```python
from build123d import *

# Parameters (mm, degrees)
SKETCH1_W                    = 42.3
SKETCH1_H                    = 42.3
BOSS_EXTRUDE1_DEPTH          = 23.5
FILLET1_R                    = 4
SKETCH2_R                    = 1.5
CUT_EXTRUDE1_DEPTH           = 5
CHAMFER1_SIZE                = 1
CIRPATTERN1_COUNT            = 4
CHAMFER1_OF_CIRPATTERN1_SIZE = 1
SKETCH3_R                    = 11
BOSS_EXTRUDE2_DEPTH          = 2
SKETCH4_R                    = 2.5
BOSS_EXTRUDE3_DEPTH          = 20
FILLET2_R                    = 1
SKETCH5_W                    = 6
SKETCH5_H                    = 16.2
BOSS_EXTRUDE4_DEPTH          = 1
SKETCH6_W                    = 1
SKETCH6_H                    = 1
BOSS_EXTRUDE5_DEPTH          = 4.5
SKETCH7_W                    = 4
SKETCH7_H                    = 4
CUT_EXTRUDE2_DEPTH           = 18


with BuildPart() as part:
    # Sketch1 → Boss-Extrude1 (new body)
    with BuildSketch(Plane.XY):
        Rectangle(SKETCH1_W, SKETCH1_H)
    extrude(amount=BOSS_EXTRUDE1_DEPTH)

    # Fillet1
    fillet1_edges = [part.edges().sort_by_distance(p)[0] for p in [
        (-21.15, 21.15, 11.75),
        (21.15, 21.15, 11.75),
        (21.15, -21.15, 11.75),
        (-21.15, -21.15, 11.75),
    ]]
    fillet(fillet1_edges, radius=FILLET1_R)

    # Sketch2 → Cut-Extrude1 (cut)
    with BuildSketch(Plane.XY.offset(23.5)):
        with Locations((-15.5, -15.5)):
            Circle(SKETCH2_R)
    cut_extrude1 = extrude(amount=-CUT_EXTRUDE1_DEPTH, mode=Mode.SUBTRACT)

    # Chamfer1
    chamfer1_edges = [part.edges().sort_by_distance(p)[0] for p in [
        (-17, -15.5, 23.5),
    ]]
    chamfer(chamfer1_edges, length=CHAMFER1_SIZE)

    # CirPattern1: Cut-Extrude1 ×4 about axis
    cirpattern1_axis = Axis((0, 0, 0), (0, 0, 1))
    for i in range(1, CIRPATTERN1_COUNT):
        add(cut_extrude1.rotate(cirpattern1_axis, i * 360 / CIRPATTERN1_COUNT), mode=Mode.SUBTRACT)

    # Chamfer1 of CirPattern1
    chamfer1_of_cirpattern1_edges = [part.edges().sort_by_distance(p)[0] for p in [
        (15.5, -17, 23.5),
        (17, 15.5, 23.5),
        (-15.5, 17, 23.5),
    ]]
    chamfer(chamfer1_of_cirpattern1_edges, length=CHAMFER1_OF_CIRPATTERN1_SIZE)

    # Sketch3 → Boss-Extrude2 (add)
    with BuildSketch(Plane.XY.offset(23.5)):
        Circle(SKETCH3_R)
    extrude(amount=BOSS_EXTRUDE2_DEPTH)

    # Sketch4 → Boss-Extrude3 (add)
    with BuildSketch(Plane.XY.offset(25.5)):
        Circle(SKETCH4_R)
    extrude(amount=BOSS_EXTRUDE3_DEPTH)

    # Fillet2
    fillet2_edges = [part.edges().sort_by_distance(p)[0] for p in [
        (-21.15, 0, 0),
        (-21.15, 0, 23.5),
        (0, 21.15, 0),
        (21.15, 0, 0),
        (0, -21.15, 0),
        (-19.978427125, -19.978427125, 0),
        (19.978427125, -19.978427125, 0),
        (19.978427125, 19.978427125, 0),
        (-19.978427125, 19.978427125, 0),
        (0, 21.15, 23.5),
        (0, -21.15, 23.5),
        (21.15, 0, 23.5),
        (-19.978427125, -19.978427125, 23.5),
        (19.978427125, -19.978427125, 23.5),
        (19.978427125, 19.978427125, 23.5),
        (-19.978427125, 19.978427125, 23.5),
        (-11, 0, 25.5),
        (-2.5, 0, 45.5),
    ]]
    fillet(fillet2_edges, radius=FILLET2_R)

    # Sketch5 → Boss-Extrude4 (add)
    with BuildSketch(Plane(origin=(21.15, 0, 0), x_dir=(0, 0, -1), z_dir=(1, 0, 0))):
        with Locations((-6.2, 0)):
            Rectangle(SKETCH5_W, SKETCH5_H)
    extrude(amount=BOSS_EXTRUDE4_DEPTH)

    # Sketch6 → Boss-Extrude5 (add)
    with BuildSketch(Plane(origin=(22.15, 0, 0), x_dir=(0, 0, -1), z_dir=(1, 0, 0))):
        Polygon((-9.2, -7.1), (-4.2, -7.1), (-4.2, 7.1), (-9.2, 7.1), (-9.2, 8.1), (-3.2, 8.1), (-3.2, -8.1), (-9.2, -8.1), align=None)
        with Locations((-6.7, -4.26)):
            Rectangle(SKETCH6_W, SKETCH6_H)
        with Locations((-6.7, 1.42)):
            Rectangle(SKETCH6_W, SKETCH6_H)
        with Locations((-6.7, 4.26)):
            Rectangle(SKETCH6_W, SKETCH6_H)
        with Locations((-6.7, -1.42)):
            Rectangle(SKETCH6_W, SKETCH6_H)
    extrude(amount=BOSS_EXTRUDE5_DEPTH)

    # Sketch7 → Cut-Extrude2 (cut)
    with BuildSketch(Plane.XY.offset(45.5)):
        with Locations((-3.5, 0)):
            Rectangle(SKETCH7_W, SKETCH7_H)
    extrude(amount=-CUT_EXTRUDE2_DEPTH, mode=Mode.SUBTRACT)


solid = part.part
```
Read the model definition and answer for the solid it produces. Units are mm, in the model's axes. A direction names the side the tool comes from. Coordinates: 2 decimals unless noted, no trailing zeros. Write each loop counter-clockwise with the first axis right and the second up, starting at its lowest first coordinate (ties: lowest second). Pieces come first, ordered by that corner, then holes. Notation, with made-up numbers: (5.5, 44) -> (23.5, 44) arc R20 ccw to (23.5, 58) -> close; hole circle Ø8 at (15.25, 44). An arc over 180 degrees is marked (long way). Answer as a JSON object with one key per item and string values.
Q1. The part is cut by section A-A on z = 21. Give the vertices of the cut face in (x, y), then the cut area to 3 significant figures.
The answers:
{"outline": "(-21.15, -17.15) arc R4 ccw to (-17.15, -21.15) -> (17.15, -21.15) arc R4 ccw to (21.15, -17.15) -> (21.15, 17.15) arc R4 ccw to (17.15, 21.15) -> (-17.15, 21.15) arc R4 ccw to (-21.15, 17.15) -> close; hole circle Ø3 at (-15.5, -15.5); hole circle Ø3 at (-15.5, 15.5); hole circle Ø3 at (15.5, -15.5); hole circle Ø3 at (15.5, 15.5)", "area": "1,750 mm2"}
Q2. The part is cut by section B-B on x = -15.5. Give the vertices of the cut face in (y, z).
The answers:
{"outline": "(-21.15, 1) arc R1 ccw to (-20.15, 0) -> (20.15, 0) arc R1 ccw to (21.15, 1) -> (21.15, 22.5) arc R1 ccw to (20.15, 23.5) -> (18, 23.5) -> (17, 22.5) -> (17, 18.5) -> (14, 18.5) -> (14, 22.5) -> (13, 23.5) -> (-13, 23.5) -> (-14, 22.5) -> (-14, 18.5) -> (-17, 18.5) -> (-17, 22.5) -> (-18, 23.5) -> (-20.15, 23.5) arc R1 ccw to (-21.15, 22.5) -> close"}
Q3. Flat-ended cylindrical pins translate along their axes: pin 1 Ø1.6 at (x, y) = (23, 3) entering from +Z; pin 2 Ø3.5 at (x, y) = (23.5, -0.5) entering from +Z; pin 3 Ø2.5 at (y, z) = (-1.5, 8) entering from +X; pin 4 Ø1.6 at (x, z) = (24.5, 5) entering from -Y. Find the tip coordinate at first contact, or state that the pin passes through.
The answers:
{"pin 1": "stops at z = 7.2", "pin 2": "stops at z = 9.2", "pin 3": "stops at x = 26.65", "pin 4": "stops at y = -8.1"}
Q4. Consider line 1 (Y direction, x = 15.5, z = 21); line 2 (X direction, y = -15, z = 20); line 3 (X direction, y = 0, z = 41). Determine where each line is inside the solid, lowest interval first. Write a range as [from, to].
The answers:
{"line 1": "y = [-21.15, -17], [-14, 14], [17, 21.15]", "line 2": "x = [-21.15, -16.91], [-14.09, 14.09], [16.91, 21.15]", "line 3": "x = [-1.5, 2.5]"}
Q5. Determine the mould class of faces 1 (the flat face through (15, -16, 18.5)), 2 (the flat face through (21.4, 0, 9.2)), 3 (the cylindrical face through (19.947, -20.009, 11.901)), 4 (the cylindrical face through (2.385, 0.751, 34.867)) for opening direction Y: pulls with the +Y half, pulls with the -Y half, needs draft (parallel to the pull), parting line crosses it, or undercut.
The answers:
{"face 1": "undercut", "face 2": "needs draft", "face 3": "pulls with the -Y half", "face 4": "parting line crosses it"}
Q6. A tool of negligible diameter and unlimited length cuts with its end or side. For faces 5 (the cylindrical face through (20.009, 19.947, 11.901)), 6 (the flat face through (24, 7.1, 7)), 7 (the flat face through (24, 0, 4.2)), 8 (the flat face through (-1.5, 0, 37)), 9 (the cylindrical face through (17, 15.43, 20.53)), from which of +Z, -Z, +X, -X, +Y, -Y can it reach the whole face along a straight path? Write none if from no direction.
The answers:
{"face 5": "+Z, -Z, +X, +Y", "face 6": "+Z, +X", "face 7": "+X", "face 8": "+Z, -X, +Y, -Y", "face 9": "+Z"}
Q7. The part is cut by section C-C on y = 12. Give the vertices of the cut face in (x, z).
The answers:
{"outline": "(-21.15, 1) arc R1 ccw to (-20.15, 0) -> (20.15, 0) arc R1 ccw to (21.15, 1) -> (21.15, 22.5) arc R1 ccw to (20.15, 23.5) -> (-20.15, 23.5) arc R1 ccw to (-21.15, 22.5) -> close"}
Q8. The part is cut by section D-D on x = 0. Give the vertices of the cut face in (y, z), then the cut area to 3 significant figures.
The answers:
{"outline": "(-21.15, 1) arc R1 ccw to (-20.15, 0) -> (20.15, 0) arc R1 ccw to (21.15, 1) -> (21.15, 22.5) arc R1 ccw to (20.15, 23.5) -> (11, 23.5) -> (11, 24.5) arc R1 ccw to (10, 25.5) -> (2.5, 25.5) -> (2.5, 44.5) arc R1 ccw to (1.5, 45.5) -> (-1.5, 45.5) arc R1 ccw to (-2.5, 44.5) -> (-2.5, 25.5) -> (-10, 25.5) arc R1 ccw to (-11, 24.5) -> (-11, 23.5) -> (-20.15, 23.5) arc R1 ccw to (-21.15, 22.5) -> close", "area": "1,140 mm2"}
